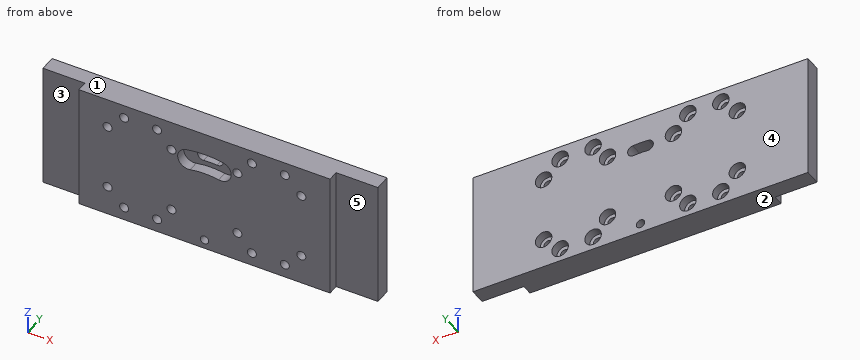
from build123d import *

# Parameters (mm, degrees)
SKETCH1_W                      = 203.2
SKETCH1_H                      = 76.2
BOSS_EXTRUDE1_DEPTH            = 15.875
F_1_4_20_TAPPED_HOLE1_D        = 5.1054
CUT_EXTRUDE1_DEPTH             = 110.663966849
CUT_EXTRUDE2_DEPTH             = 6.35
CBORE_FOR_M5_SHCS2_D           = 5.5
CBORE_FOR_M5_SHCS2_CBORE_D     = 10
CBORE_FOR_M5_SHCS2_CBORE_DEPTH = 5.1
SKETCH12_W                     = 25.4
SKETCH12_H                     = 76.2
CUT_EXTRUDE3_DEPTH             = 6.35


with BuildPart() as part:
    # Sketch1 → Boss-Extrude1 (new body)
    with BuildSketch(Plane(origin=(0, 0, 0), x_dir=(1, 0, 0), z_dir=(0, 1, 0))):
        Rectangle(SKETCH1_W, SKETCH1_H)
    extrude(amount=BOSS_EXTRUDE1_DEPTH)

    # 1/4-20 Tapped Hole1 (through all)
    with Locations(Plane(origin=(0, 15.875, 0), x_dir=(1, 0, 0), z_dir=(0, 1, 0))):
        with Locations((0, 32.5)):
            Hole(F_1_4_20_TAPPED_HOLE1_D / 2)

    # Sketch4 → Cut-Extrude1 (cut, through all)
    with BuildSketch(Plane(origin=(0, 15.875, 0), x_dir=(1, 0, 0), z_dir=(0, 1, 0))):
        with BuildLine():
            ThreePointArc((-4.721526183, -21.467291215), (0, -21.6734375), (4.721526183, -21.467291215))
            ThreePointArc((4.721526183, -21.467291215), (7.788112283, -17.812676212), (4.133497281, -14.746090111))
            ThreePointArc((4.133497281, -14.746090111), (0, -14.9265625), (-4.133497281, -14.746090111))
            ThreePointArc((-4.133497281, -14.746090111), (-7.788112283, -17.812676212), (-4.721526183, -21.467291215))
        make_face()
    extrude(amount=-CUT_EXTRUDE1_DEPTH, mode=Mode.SUBTRACT)

    # Sketch6 → Cut-Extrude2 (cut)
    with BuildSketch(Plane.XZ):
        with BuildLine():
            ThreePointArc((11.149411903, 23.551878775), (0, 24.65), (-11.149411903, 23.551878775))
            ThreePointArc((-11.149411903, 23.551878775), (-16.138574889, 16.0850687), (-8.671764814, 11.095905714))
            ThreePointArc((-8.671764814, 11.095905714), (0, 11.95), (8.671764814, 11.095905714))
            ThreePointArc((8.671764814, 11.095905714), (16.138574889, 16.0850687), (11.149411903, 23.551878775))
        make_face()
    extrude(amount=-CUT_EXTRUDE2_DEPTH, mode=Mode.SUBTRACT)

    # CBORE for M5 SHCS2 (through all)
    with Locations(Plane(origin=(0, 15.875, 0), x_dir=(1, 0, 0), z_dir=(0, 1, 0))):
        with Locations((58.76, -20), (48.755, -30), (28.755, -30), (20, -20), (20, 20), (28.755, 30), (48.755, 30), (58.76, 20), (-28.755, 30), (-20, 20), (-48.755, 30), (-58.76, 20), (-58.76, -20), (-48.755, -30), (-28.755, -30), (-20, -20)):
            CounterBoreHole(CBORE_FOR_M5_SHCS2_D / 2, CBORE_FOR_M5_SHCS2_CBORE_D / 2, CBORE_FOR_M5_SHCS2_CBORE_DEPTH)

    # Sketch12 → Cut-Extrude3 (cut)
    with BuildSketch(Plane.XZ):
        with Locations((88.9, 0)):
            Rectangle(SKETCH12_W, SKETCH12_H)
    cut_extrude3 = extrude(amount=-CUT_EXTRUDE3_DEPTH, mode=Mode.SUBTRACT)

    # Mirror1: Cut-Extrude3 across plane
    add(cut_extrude3.mirror(Plane(origin=(0, 0, 0), x_dir=(0, 0, 1), z_dir=(1, 0, 0))), mode=Mode.SUBTRACT)


solid = part.part
The model under review builds one solid part; all positions refer to its coordinate system, in mm. Face numbers are marked on the shaded views. A direction names the side the tool comes from. Round coordinates to 2 decimals unless told otherwise and drop trailing zeros. Loops run counter-clockwise (first coordinate to the right, second up) from the corner with the lowest first, then second, coordinate; pieces in that order, holes last. Notation, with made-up numbers: (47, 38) -> (103, 38) arc R22 ccw to (103, 55) -> close; hole circle Ø1 at (-25, 83.5). An arc over 180 degrees is marked (long way). One line per question, with ' | ' between items. Start each with the question number.
Item 1: Wall thickness on line 1 along Z through (x, y) = (-58.76, 2.75); line 2 along Z through (x, y) = (20, 14.6); line 3 along X through (y, z) = (13.1, -20): over which ranges is each line inside the solid? List them lowest first. Write a range as [from, to].
Item 2: Draft analysis for pull direction Z (two halves, no side actions). For the marked faces 1, 2 and 3, state which applies: +Z half, -Z half, draft (parallel to the pull), parting line (faces both ways), or undercut.
Item 3: Add section B-B, the plane y = 8.75. Count the separate pieces of the cut face and the enclosed holes in it, then the cut area to 3 significant figures.
Item 4: Machinability: for the marked faces 4 and 5, which of the approach directions +Z, -Z, +X, -X, +Y, -Y give a long, thin tool a straight path to every point of the face, cutting with its end or side? Answer none if there is none.
Item 5: Add section D-D, the plane z = -1. Write out the cut boundary in (x, y) (3 decimals), then the cut area to 3 significant figures.
Item 6: Add section A-A, the plane x = -20. Write out the cut boundary in (y, z) (3 decimals), then the cut area to 3 significant figures.
Item 7: For pin 1 (7 mm diameter, centred on y = 3, z = 4, fed in from -X); pin 2 (3 mm diameter, centred on y = 3, z = -16, fed in from -X); pin 3 (7 mm diameter, centred on x = 20, z = 20, fed in from +Y) (3 decimals); pin 4 (20.5 mm diameter, centred on x = 87, z = 11.5, fed in from -Y), all flat-tipped, find the tip position at first contact; note any pin that passes through.
Return value:
1) line 1: z = [-38.1, -22.75], [-17.25, 17.25], [22.75, 38.1] | line 2: z = [-38.1, -25], [-15, 15], [25, 38.1] | line 3: x = [-101.6, -63.76], [-53.76, -25], [-15, 15], [25, 53.76], [63.76, 101.6]
2) face 1: +Z half | face 2: -Z half | face 3: draft
3) separate pieces: 1 | enclosed holes: 18 | area: 15,000 mm2
4) face 4: +Z, -Z, +X, -X, +Y | face 5: +Z, -Z, +X, -Y
5) outline: (-101.6, 6.35) -> (-76.2, 6.35) -> (-76.2, 0) -> (76.2, 0) -> (76.2, 6.35) -> (101.6, 6.35) -> (101.6, 15.875) -> (-101.6, 15.875) -> close | area: 2,900 mm2
6) outline: (0, -38.1) -> (15.875, -38.1) -> (15.875, -25) -> (10.775, -25) -> (10.775, -22.75) -> (0, -22.75) -> close; (0, -17.25) -> (10.775, -17.25) -> (10.775, -15) -> (15.875, -15) -> (15.875, 15) -> (10.775, 15) -> (10.775, 17.25) -> (0, 17.25) -> close; (0, 22.75) -> (10.775, 22.75) -> (10.775, 25) -> (15.875, 25) -> (15.875, 38.1) -> (0, 38.1) -> close | area: 989 mm2
7) pin 1: stops at x = -101.6 | pin 2: stops at x = -76.2 | pin 3: stops at y = 10.775 | pin 4: stops at y = 6.35
